Read the model definition and answer for the solid it produces. Units are mm, in the model's axes. A direction names the side the tool comes from. Give positions to 0.01 mm unless a question says otherwise; leave off trailing zeros. Order: outer loops, then holes, each group sorted by start corner. A loop starts at its lowest first (then second) coordinate and runs counter-clockwise, first axis right, second up. Notation, with made-up numbers: (8, -37.75) - (41, -37.75) arc R11 cw to (41, -17.75) - close; hole circle Ø2 at (66, 49.5). An arc over 180 degrees is marked (long way). One line per item, written item: value. Start each with the question number.
```python
from build123d import *

# Parameters (mm, degrees)
F1_DEPTH = 5.08
F2_SIZE  = 2.53999


# Not quite as in the source:
# - a fillet or chamfer is up to 0.001 mm smaller than in the source, because OpenCascade refuses the exact size


with BuildPart() as f1:
    # F0 (on Top) → F1 (new body)
    with BuildSketch(Plane.XY):
        Polygon((0, 0), (0, 72.3038464785), (-11.8312668055, 48.0264090002), (-7.1868877858, 36.4154614508), (-13.0979157984, 21.6378867626), (-6.9757793099, 2.6381509379), (-16.4937096578, -0.428737424), align=None)
    extrude(amount=F1_DEPTH)

    # F2 (size 2.54 in the source; OpenCascade refuses exactly that, so slightly less here)
    f2_edges = [f1.edges().sort_by_distance(p)[0] for p in [
        (-5.915633, 60.165128, 5.08),
        (-9.509077, 42.220935, 5.08),
        (-10.142402, 29.026674, 5.08),
        (-10.036848, 12.138019, 5.08),
        (-11.734744, 1.104707, 5.08),
        (-5.915633, 60.165128, 0),
        (-9.509077, 42.220935, 0),
        (-10.142402, 29.026674, 0),
        (-10.036848, 12.138019, 0),
        (-11.734744, 1.104707, 0),
    ]]
    chamfer(f2_edges, length=F2_SIZE)


solid = f1.part
```
1) Find the intervals of material crossed by probe 1 along Y at (x, z) = (-2.25, 4.45); probe 2 along X at (y, z) = (68, 1.3); probe 3 along Y at (x, z) = (-5.5, 1.85), in increasing order. Write a range as from..to.
2) For faces 5 (the flat face through (-4.675, 59.771, 3.828)), 6 (the flat face through (-8.16, 42.32, 1.25)), 7 (the flat face through (-8.47, 11.474, 3.828)), determine the directions among +Z, -Z, +X, -X, +Y, -Y from which every point of the face is accessible in a straight line to the end or side of a thin tool.
3) Section A-A on x = -8.25 is taken. Give the number of separate pieces and of enclosed holes in the cut face, plus the area to 3 significant figures.
4) Section B-B on z = 1.8 is taken. Write down the section's boundary in (x, y), plus the area to 3 significant figures.
5) The mould has two halves that part along Y. Classify faces 1 (the flat face through (-8.71, 29.13, 1.25)), 2 (the flat face through (-4.675, 59.771, 1.252)), 3 (the flat face through (-8.71, 29.13, 3.83)), 4 (the flat face through (0, 36, 3)): +Y half, -Y half, draft (parallel to the pull), parting line (faces both ways), or undercut.
6) Each of these flat-tipped pins is pushed along its axis until it touches: pin 1 (1.5 mm diameter, centred on y = 58.5, z = 2.5, fed in from -X); pin 2 (1.5 mm diameter, centred on y = 14.5, z = 3.5, fed in from -X). Where does it stop, or does it pass through?
Solved:
1. probe 1: y = -0.06..63.33
1. probe 2: x = -0.72..0
1. probe 3: y = -0.14..59.44
2. face 5: +Z, -X, +Y
2. face 6: -Z, -X
2. face 7: +Z, -X
3. separate pieces: 3
3. enclosed holes: 0
3. area: 156 mm2
4. outline: (-13.87, -0.36) - (0, 0) - (0, 70.61) - (-11.02, 48) - (-6.39, 36.42) - (-12.31, 21.61) - (-6.04, 2.16) - close
4. area: 565 mm2
5. face 1: undercut
5. face 2: +Y half
5. face 3: undercut
5. face 4: draft
6. pin 1: stops at x = -7.09
6. pin 2: stops at x = -10.61
